from build123d import *

# Parameters (mm, degrees)
SKETCH1_R      = 5
EXTRUDE1_DEPTH = 3.94
HOLE1_D        = 7.996833333
HOLE1_DEPTH    = 0.656666667
SKETCH4_R      = 2.748625
EXTRUDE2_DEPTH = 0.656666667
HOLE2_D        = 7.996833333
HOLE2_DEPTH    = 0.656666667
SKETCH7_R      = 2.748625
EXTRUDE3_DEPTH = 0.656666667
HOLE3_D        = 3.9975
HOLE3_DEPTH    = 3.94
CHAMFER1_SIZE  = 0.197


with BuildPart() as part:
    # Sketch1 → Extrude1 (new body)
    with BuildSketch(Plane.XY.offset(3.94)):
        Circle(SKETCH1_R)
    extrude(amount=-EXTRUDE1_DEPTH)

    # Hole1
    with Locations(Plane.XY.offset(3.94)):
        with Locations((0, 0)):
            Hole(HOLE1_D / 2, depth=HOLE1_DEPTH)

    # Sketch4 → Extrude2 (add)
    with BuildSketch(Plane.XY.offset(3.283333333)):
        Circle(SKETCH4_R)
    extrude(amount=EXTRUDE2_DEPTH)

    # Hole2
    with Locations(Plane(origin=(0, 0, 0), x_dir=(-1, 0, 0), z_dir=(0, 0, -1))):
        with Locations((0, 0)):
            Hole(HOLE2_D / 2, depth=HOLE2_DEPTH)

    # Sketch7 → Extrude3 (add)
    with BuildSketch(Plane(origin=(0, 0, 0.656666667), x_dir=(-1, 0, 0), z_dir=(0, 0, -1))):
        Circle(SKETCH7_R)
    extrude(amount=EXTRUDE3_DEPTH)

    # Hole3
    with Locations(Plane(origin=(0, 0, 0), x_dir=(-1, 0, 0), z_dir=(0, 0, -1))):
        with Locations((0, 0)):
            Hole(HOLE3_D / 2, depth=HOLE3_DEPTH)

    # Chamfer1
    chamfer1_edges = [part.edges().sort_by_distance(p)[0] for p in [
        (-5, 0, 3.94),
        (-1.99875, 0, 0),
        (-1.99875, 0, 3.94),
        (-5, 0, 0),
    ]]
    chamfer(chamfer1_edges, length=CHAMFER1_SIZE)


solid = part.part
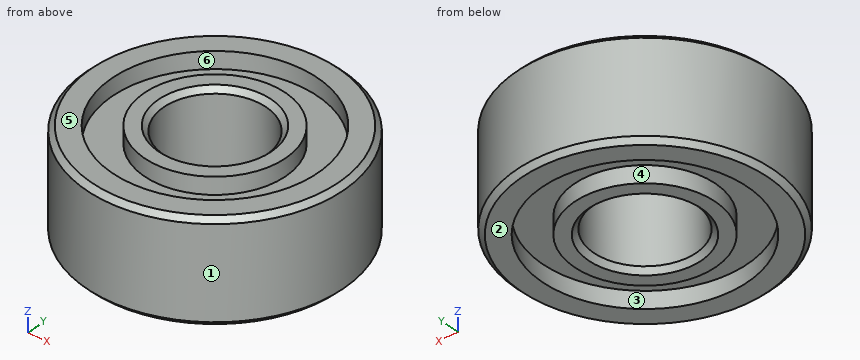
Work out the finished part from the listing and answer in its coordinate system (mm). Face numbers are marked on the shaded views. A direction names the side the tool comes from. Round coordinates to 2 decimals unless told otherwise and drop trailing zeros. Write each loop counter-clockwise with the first axis right and the second up, starting at its lowest first coordinate (ties: lowest second). Pieces come first, ordered by that corner, then holes.
1) A cutting plane is placed at B-B (z = 1.1). Give the vertices of the cut face in (x, y).
2) Straight lines are drawn through the part: line 1 (Y direction, x = 0, z = 0.45); line 2 (Y direction, x = 0, z = 2.2); line 3 (X direction, y = -0.25, z = 0.35). For each, find the intervals that lie inside material, in ascending order.
3) A tool of negligible diameter and unlimited length cuts with its end or side. For the marked faces 4, 5 and 6, from which of +Z, -Z, +X, -X, +Y, -Y can it reach the whole face along a straight path? Write none if from no direction.
4) A cutting plane is placed at C-C (z = 3.45). Give the vertices of the cut face in (x, y).
5) The mould has two halves that part along Y. Classify the marked faces 1, 2 and 3: pulls with the +Y half, pulls with the -Y half, needs draft (parallel to the pull), parting line crosses it, or undercut.
6) Given pin 1 Ø1 at (x, z) = (-2.5, 1) entering from -Y; pin 2 Ø2 at (x, z) = (1.5, 1) entering from -Y, each flat-ended and moving along its own axis, determine where each tip first touches the part or whether it passes through.
Completed:
1. outline: circle Ø10 at (0, 0); hole circle Ø4 at (0, 0)
2. line 1: y = -5 to -4, -2.75 to -2, 2 to 2.75, 4 to 5
2. line 2: y = -5 to -2, 2 to 5
2. line 3: x = -4.99 to -3.99, -2.74 to -1.98, 1.98 to 2.74, 3.99 to 4.99
3. face 4: -Z
3. face 5: +Z, +X, -X, +Y, -Y
3. face 6: +Z
4. outline: circle Ø10 at (0, 0); circle Ø5.5 at (0, 0); hole circle Ø8 at (0, 0); hole circle Ø4 at (0, 0)
5. face 1: parting line crosses it
5. face 2: needs draft
5. face 3: undercut
6. pin 1: stops at y = -4.58
6. pin 2: stops at y = -4.97
